```python
from build123d import *

# Parameters (mm, degrees)
SKETCH_2_W          = 2.54
SKETCH_2_H          = 2.54
EXTRUDE_1_DEPTH     = 8.5
SKETCH_3_W          = 0.3
SKETCH_3_H          = 0.5
EXTRUDE_2_DEPTH     = 3.96
SKETCH_4_W          = 1.5
SKETCH_4_H          = 1.5
CUT_EXTRUDE_1_DEPTH = 7


with BuildPart() as part:
    # 草图2 → 拉伸1 (new body)
    with BuildSketch(Plane(origin=(0, 0, 0), x_dir=(1, 0, 0), z_dir=(0, 1, 0))):
        Rectangle(SKETCH_2_W, SKETCH_2_H)
    extrude(amount=EXTRUDE_1_DEPTH)

    # 草图3 → 拉伸2 (add)
    with BuildSketch(Plane.XZ):
        Rectangle(SKETCH_3_W, SKETCH_3_H)
    extrude(amount=EXTRUDE_2_DEPTH)

    # 草图4 → 切除-拉伸1 (cut)
    with BuildSketch(Plane(origin=(0, 8.5, 0), x_dir=(-1, 0, 0), z_dir=(0, 1, 0))):
        Rectangle(SKETCH_4_W, SKETCH_4_H)
    extrude(amount=-CUT_EXTRUDE_1_DEPTH, mode=Mode.SUBTRACT)


solid = part.part
```
Check sheet for the modelled part. Datum: model origin and axes. Units: mm. A direction names the side the tool comes from. Coordinates: 2 decimals unless noted, no trailing zeros. Loops run counter-clockwise (first coordinate to the right, second up) from the corner with the lowest first, then second, coordinate; pieces in that order, holes last. Notation, with made-up numbers: M 82.25,37.25 L 129.25,37.25 A25 cw 129.25,74.25 Z; hole C 53,-30 d4. An arc over 180 degrees is marked long. Answer as a JSON object with one key per item and string values.
1. Sectioned sample at B-B on y = 7.5. Record the cut outline in (x, z), and give its area (3 significant figures).
Outcome:
{"outline": "M -1.27,-1.27 L 1.27,-1.27 L 1.27,1.27 L -1.27,1.27 Z; hole M -0.75,-0.75 L 0.75,-0.75 L 0.75,0.75 L -0.75,0.75 Z", "area": "4.20 mm²"}
2. Release check for a two-part mould opening along Z. For faces 1 (the flat face through (0, 5, 0.75)), 2 (the flat face through (0.3, 0, -0.3)), 3 (the flat face through (0, 4, -1.27)) record: pulls with the +Z half, pulls with the -Z half, needs draft (parallel to the pull), parting line crosses it, or undercut.
Outcome:
{"face 1": "undercut", "face 2": "needs draft", "face 3": "pulls with the -Z half"}
3. Sectioned sample at A-A on z = -0.4. Record the cut outline in (x, y), and give its area (3 significant figures).
Outcome:
{"outline": "M -1.27,0 L 1.27,0 L 1.27,8.5 L 0.75,8.5 L 0.75,1.5 L -0.75,1.5 L -0.75,8.5 L -1.27,8.5 Z", "area": "11.1 mm²"}
4. Access from +Z, -Z, +X, -X, +Y, -Y to the whole of each face (thin tool, end or side, straight path). Record for faces 4 (the flat face through (0, 8.5, -1)), 5 (the flat face through (0.75, 5, 0)).
Outcome:
{"face 4": "+Z, -Z, +X, -X, +Y", "face 5": "+Y"}
5. Scan lines: L1, parallel to Z at x = -0.35, y = 5.75; L2, parallel to Y at x = -0.95, z = 0.55. Record each from-to range of solid material in increasing order. Write a range as from..to.
Outcome:
{"L1": "-1.27..-0.75, 0.75..1.27", "L2": "0..8.5"}
6. Sectioned sample at C-C on x = -0.6. Record the cut outline in (y, z).
Outcome:
{"outline": "M 0,-1.27 L 8.5,-1.27 L 8.5,-0.75 L 1.5,-0.75 L 1.5,0.75 L 8.5,0.75 L 8.5,1.27 L 0,1.27 Z"}
7. Sectioned sample at D-D on y = -2.25. Record the cut outline in (x, z), and give its area (3 significant figures).
Outcome:
{"outline": "M -0.15,-0.25 L 0.15,-0.25 L 0.15,0.25 L -0.15,0.25 Z", "area": "0.150 mm²"}
